Verification items for the finished model (mm, model axes). Face numbers are marked on the shaded views. A direction names the side the tool comes from. Give positions to 0.01 mm unless a question says otherwise; leave off trailing zeros. Loops run counter-clockwise (first coordinate to the right, second up) from the corner with the lowest first, then second, coordinate; pieces in that order, holes last. Notation, with made-up numbers: (58.25, 61.25) -> (115.25, 61.25) arc R23 cw to (115.25, 82.25) -> close; hole circle Ø3 at (8, 79.25). An arc over 180 degrees is marked (long way). Answer in a Markdown table with one row per item. Add a question column.
Q1. Set-up check for the marked faces 1 and 2: record each of +Z, -Z, +X, -X, +Y, -Y from which the full face is reachable in a straight line by a thin tool's end or side.
Q2. Section check B-B on x = -34.5. Enter the section's corners in (y, z).
Q3. Section check A-A on y = -21.5. Enter the section's corners in (x, z), and give its area (3 significant figures).
Q4. Release check for a two-part mould opening along Y. For the marked faces 3, 4 and 5 record: pulls with the +Y half, pulls with the -Y half, needs draft (parallel to the pull), parting line crosses it, or undercut.
Q5. Section check C-C on z = 1.5. Give the number of separate pieces and of enclosed holes in the cut face, and give its area (3 significant figures).
Q6. Section check D-D on y = -5.5. Enter the section's corners in (x, z), and give its area (3 significant figures).
Q7. Gauge pin test, flat ends, axial feed: P1, Ø1.5, axis at y = 29, z = 6, coming from the +X side; P2, Ø1.5, axis at y = 39, z = 4, coming from the +X side; P3, Ø3.5, axis at x = 3, z = 2, coming from the -Y side; P4, Ø6, axis at x = -16.5, y = 9, coming from the -Z side. Record the tip position at first contact, or that the pin passes through.
Q8. Material ranges on probe 1 along X at (y, z) = (-14, 2); probe 2 along X at (y, z) = (16, 6.75); probe 3 along Y at (x, z) = (-16.5, 1.5), recorded low to high.
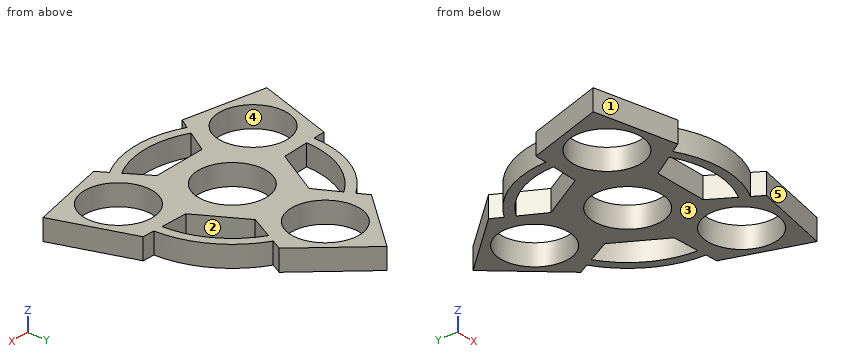
```python
from build123d import *

# Parameters (mm, degrees)
F0_R     = 11.10107
F1_DEPTH = 6.9342
F3_DEPTH = 6.9342


with BuildPart() as f1:
    # F0 (on Top) → F1 (new body)
    with BuildSketch(Plane.XY):
        Polygon((18.1369372315, 30.5542092799), (0, 50.8), (-18.1369372315, 30.5542092799), (-10.5741708498, 16.3638919404), (-19.4586315501, 0.9755546097), (-35.5291900447, 0.4299437494), (-43.9940905122, -25.4), (-17.3922528132, -30.9841530293), (-8.8844607003, -17.3394465501), (8.8844607003, -17.3394465501), (17.3922528132, -30.9841530293), (43.9940905122, -25.4), (35.5291900447, 0.4299437494), (19.4586315501, 0.9755546097), (10.5741708498, 16.3638919404), align=None)
        with Locations((-26.4607214289, -15.27710464)):
            Circle(F0_R, mode=Mode.SUBTRACT)
        with Locations((26.4607214289, -15.27710464)):
            Circle(F0_R, mode=Mode.SUBTRACT)
        Circle(F0_R, mode=Mode.SUBTRACT)
        with Locations((0, 30.5542092799)):
            Circle(F0_R, mode=Mode.SUBTRACT)
    extrude(amount=F1_DEPTH)

    # F2 (on face) → F3 (join)
    with BuildSketch(Plane.XY.offset(6.9342)):
        with BuildLine():
            Line((15.2522996768, -27.5521189554), (13.6293113813, -24.9491875935))
            ThreePointArc((13.6293113813, -24.9491875935), (0, -28.4292119185), (-13.6293113813, -24.9491875935))
            Line((-13.6293113813, -24.9491875935), (-15.2522996768, -27.5521189554))
            ThreePointArc((-15.2522996768, -27.5521189554), (0, -31.4920927276), (15.2522996768, -27.5521189554))
        make_face()
        with BuildLine():
            ThreePointArc((14.7919745691, 24.2779236891), (24.620419731, 14.2146059592), (28.4212859504, 0.6712639045))
            Line((28.4212859504, 0.6712639045), (31.4869847819, 0.5671804915))
            ThreePointArc((31.4869847819, 0.5671804915), (27.2729523205, 15.7460463638), (16.2346851051, 26.984938464))
            Line((16.2346851051, 26.984938464), (14.7919745691, 24.2779236891))
        make_face()
        with BuildLine():
            ThreePointArc((-28.4212859504, 0.6712639045), (-24.620419731, 14.2146059592), (-14.7919745691, 24.2779236891))
            Line((-14.7919745691, 24.2779236891), (-16.2346851051, 26.984938464))
            ThreePointArc((-16.2346851051, 26.984938464), (-27.2729523205, 15.7460463638), (-31.4869847819, 0.5671804915))
            Line((-31.4869847819, 0.5671804915), (-28.4212859504, 0.6712639045))
        make_face()
    extrude(amount=-F3_DEPTH)


solid = f1.part
```
Taken from the geometry:
| question | item | result |
|---|---|---|
| 1 | face 1 | +Z, -Z, -X, -Y |
| 1 | face 2 | +Z, -Z |
| 2 | outline | (-27.39, 0) -> (-22.93, 0) -> (-22.93, 6.93) -> (-27.39, 6.93) -> close; (-7.62, 0) -> (0.46, 0) -> (0.46, 6.93) -> (-7.62, 6.93) -> close |
| 3 | outline | (-42.72, 0) -> (-35.65, 0) -> (-35.65, 6.93) -> (-42.72, 6.93) -> close; (-17.27, 0) -> (-11.48, 0) -> (-11.48, 6.93) -> (-17.27, 6.93) -> close; (11.48, 0) -> (17.27, 0) -> (17.27, 6.93) -> (11.48, 6.93) -> close; (35.65, 0) -> (42.72, 0) -> (42.72, 6.93) -> (35.65, 6.93) -> close |
| 3 | area | 178 mm² |
| 4 | face 3 | needs draft |
| 4 | face 4 | undercut |
| 4 | face 5 | pulls with the -Y half |
| 5 | separate pieces | 1 |
| 5 | enclosed holes | 7 |
| 5 | area | 2,030 mm² |
| 6 | outline | (-37.47, 0) -> (-31.72, 0) -> (-31.72, 6.93) -> (-37.47, 6.93) -> close; (-21.2, 0) -> (-9.64, 0) -> (-9.64, 6.93) -> (-21.2, 6.93) -> close; (9.64, 0) -> (21.2, 0) -> (21.2, 6.93) -> (9.64, 6.93) -> close; (31.72, 0) -> (37.47, 0) -> (37.47, 6.93) -> (31.72, 6.93) -> close |
| 6 | area | 240 mm² |
| 7 | P1 | stops at x = 17.71 |
| 7 | P2 | stops at x = 11.24 |
| 7 | P3 | stops at y = -31.47 |
| 7 | P4 | stops at z = 0 |
| 8 | probe 1 | x = -40.26 to -37.49, -15.43 to 15.43, 37.49 to 40.26 |
| 8 | probe 2 | x = -27.12 to -23.5, -10.78 to 10.78, 23.5 to 27.12 |
| 8 | probe 3 | y = -29.55 to -20.18, -10.38 to 6.1, 23.15 to 26.82, 27.48 to 32.38 |
